Check sheet for the modelled part. Datum: model origin and axes. Units: mm. Face numbers are marked on the shaded views. A direction names the side the tool comes from. Round coordinates to 2 decimals unless told otherwise and drop trailing zeros. Order: outer loops, then holes, each group sorted by start corner. A loop starts at its lowest first (then second) coordinate and runs counter-clockwise, first axis right, second up. Notation, with made-up numbers: (10, 26.5) -> (34, 26.5) arc R19 ccw to (34, 37.5) -> close; hole circle Ø10 at (-32, 57). An arc over 180 degrees is marked (long way). Answer in a Markdown table with one row per item.
```python
from build123d import *

# Parameters (mm, degrees)
SKETCH_W      = 340.51875
SKETCH_H      = 150.01875
SKETCH_R      = 9.525
SKETCH_W_2    = 19.05
SKETCH_H_2    = 19.05
SKETCH_W_3    = 76.2
EXTRUDE_DEPTH = 25.4


with BuildPart() as part:
    # Sketch → Extrude (new body)
    with BuildSketch(Plane.XY):
        Rectangle(SKETCH_W, SKETCH_H)
        with Locations((146.446875, 51.196875)):
            Circle(SKETCH_R, mode=Mode.SUBTRACT)
        with Locations((-146.446875, 51.196875)):
            Rectangle(SKETCH_W_2, SKETCH_H_2, mode=Mode.SUBTRACT)
        Polygon((155.971875, -67.865625), (98.821875, -67.865625), (98.821875, -48.815625), (117.871875, -48.815625), (117.871875, -29.765625), (136.921875, -29.765625), (136.921875, -48.815625), (155.971875, -48.815625), align=None, mode=Mode.SUBTRACT)
        Polygon((-155.971875, -60.721875), (-155.971875, 34.528125), (129.778125, 34.528125), (129.778125, -22.621875), (110.728125, -22.621875), (110.728125, -41.671875), (91.678125, -41.671875), (91.678125, -60.721875), align=None, mode=Mode.SUBTRACT)
        with Locations((91.678125, 51.196875)):
            Rectangle(SKETCH_W_3, SKETCH_H_2, mode=Mode.SUBTRACT)
        with Locations((1.190625, 51.196875)):
            Rectangle(SKETCH_W_3, SKETCH_H_2, mode=Mode.SUBTRACT)
        with Locations((-89.296875, 51.196875)):
            Rectangle(SKETCH_W_3, SKETCH_H_2, mode=Mode.SUBTRACT)
    extrude(amount=EXTRUDE_DEPTH)


solid = part.part
```
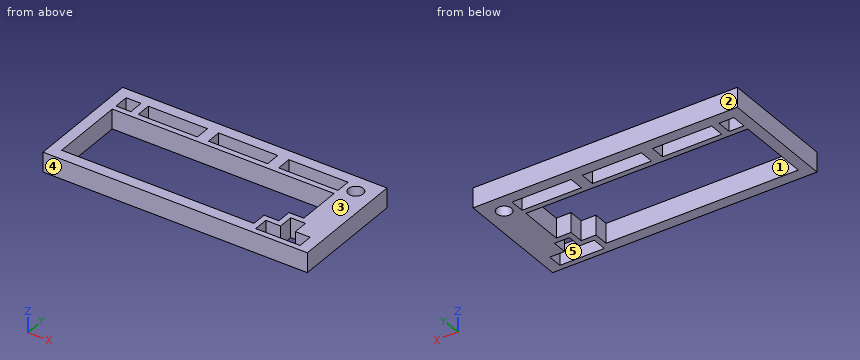
(1) Draft check along Y on the marked faces 3, 4 and 5. Enter one of: pulls with the +Y half, pulls with the -Y half, needs draft (parallel to the pull), parting line crosses it, or undercut.
Solutions:
| item | result |
|---|---|
| face 3 | needs draft |
| face 4 | pulls with the -Y half |
| face 5 | undercut |
(2) Scan lines: probe 1 along Y at (x, z) = (-2, 9.5); probe 2 along X at (y, z) = (-54.5, 17.5); probe 3 along Y at (x, z) = (109, 20.5). Record each from-to range of solid material in increasing order. Write a range as from..to.
Solutions:
| item | result |
|---|---|
| probe 1 | -75.01..-60.72, 34.53..41.67, 60.72..75.01 |
| probe 2 | -170.26..-155.97, 91.68..98.82, 155.97..170.26 |
| probe 3 | -75.01..-67.87, -48.82..-41.67, 34.53..41.67, 60.72..75.01 |
(3) Section check A-A on y = 7.5. Record the boundary of the cut face in (x, z).
Solutions:
| item | result |
|---|---|
| outline | (-170.26, 0) -> (-155.97, 0) -> (-155.97, 25.4) -> (-170.26, 25.4) -> close; (129.78, 0) -> (170.26, 0) -> (170.26, 25.4) -> (129.78, 25.4) -> close |
(4) Depth check by flat-ended pin: pin 1 Ø15 at (x, y) = (146.45, 51.2) entering from +Z. Enter the tip coordinate at first touch or a pass-through.
Solutions:
| item | result |
|---|---|
| pin 1 | through |
(5) Section check B-B on x = 15. Record the boundary of the cut face in (y, z), plus the area to 3 significant figures.
Solutions:
| item | result |
|---|---|
| outline | (-75.01, 0) -> (-60.72, 0) -> (-60.72, 25.4) -> (-75.01, 25.4) -> close; (34.53, 0) -> (41.67, 0) -> (41.67, 25.4) -> (34.53, 25.4) -> close; (60.72, 0) -> (75.01, 0) -> (75.01, 25.4) -> (60.72, 25.4) -> close |
| area | 907 mm^2 |
(6) Section check C-C on z = 19.75. Give the number of separate pieces and of enclosed holes in the cut face, plus the area to 3 significant figures.
Solutions:
| item | result |
|---|---|
| separate pieces | 1 |
| enclosed holes | 7 |
| area | 18,500 mm^2 |
(7) Tool access check on the marked faces 1 and 2. Record the directions out of +Z, -Z, +X, -X, +Y, -Y that give a thin tool (end or side, any length) a straight path to the whole face; none if there is none.
Solutions:
| item | result |
|---|---|
| face 1 | +Z, -Z |
| face 2 | +Z, -Z, +X, -X, +Y |
